```python
from build123d import *

# Parameters (mm, degrees)
F1_DEPTH    = 10
F2_R        = 1.5
F3_DEPTH    = 67.201
F5_DEPTH    = 1
F6_D        = 3.2
F7_R        = 4
F8_T1_DEPTH = 10


# Not quite as in the source:
# - a fillet or chamfer that OpenCascade refuses, or shapes differently, is made with other operations: its cross-section is extruded or revolved along the edge and cut away or added


with BuildPart() as f1:
    # F0 (on Front) → F1 (new body)
    with BuildSketch(Plane.XZ):
        with BuildLine():
            ThreePointArc((1, 29.5831032855), (0, -29.6), (-1, 29.5831032855))
            Line((-1, 29.5831032855), (-1, 41.225893517))
            Line((-1, 41.225893517), (-5, 41.225893517))
            Line((-5, 41.225893517), (-5, 33.225893517))
            ThreePointArc((-5, 33.225893517), (-19.3012329429, 27.503134492), (-29.5458965002, 16))
            Line((-29.5458965002, 16), (-33.6, 16))
            Line((-33.6, 16), (-33.6, -16))
            Line((-33.6, -16), (-29.5458965002, -16))
            ThreePointArc((-29.5458965002, -16), (0, -33.6), (29.5458965002, -16))
            Line((29.5458965002, -16), (33.6, -16))
            Line((33.6, -16), (33.6, 16))
            Line((33.6, 16), (29.5458965002, 16))
            ThreePointArc((29.5458965002, 16), (19.3012329429, 27.503134492), (5, 33.225893517))
            Line((5, 33.225893517), (5, 41.225893517))
            Line((5, 41.225893517), (1, 41.225893517))
            Line((1, 41.225893517), (1, 29.5831032855))
        make_face()
    extrude(amount=F1_DEPTH)

    # F2 (on face) → F3 (cut, through all)
    with BuildSketch(Plane.YZ.offset(33.6)):
        with Locations((-5, 10)):
            Circle(F2_R)
        with Locations((-5, -10)):
            Circle(F2_R)
    extrude(amount=-F3_DEPTH, mode=Mode.SUBTRACT)

    # F4 (on face) → F5 (cut)
    with BuildSketch(Plane.YZ.offset(5)):
        Polygon((-1.7091034656, 37.225893517), (-3.3545517328, 40.075893517), (-6.6454482672, 40.075893517), (-8.2908965344, 37.225893517), (-6.6454482672, 34.375893517), (-3.3545517328, 34.375893517), align=None)
    extrude(amount=-F5_DEPTH, mode=Mode.SUBTRACT)

    # F6 (through all)
    with Locations(Plane.YZ.offset(5)):
        with Locations((-5, 37.225893517)):
            Hole(F6_D / 2)

    # F7
    f7_edges = [f1.edges().sort_by_distance(p)[0] for p in [
        (3, 0, 41.225894),
        (3, -10, 41.225894),
        (-3, -10, 41.225894),
        (-3, 0, 41.225894),
    ]]
    fillet(f7_edges, radius=F7_R)

    # F8: chamfer of 1 on 2 edges, made by hand

    # F8_s2 → F8_t1 (join)
    with BuildSketch(Plane.XZ):
        with BuildLine():
            Line((4.9743446923, 34.2419704201), (5.9814730887, 33.0372447854))
            Line((5.9814730887, 33.0372447854), (5.977927959, 33.0175614916))
            ThreePointArc((5.977927959, 33.0175614916), (5.4901701774, 33.1281516451), (4.9970238095, 33.2061161994))
            Line((4.9970238095, 33.2061161994), (4.98, 33.225893517))
            ThreePointArc((4.98, 33.225893517), (4.98, 33.7339319685), (4.9543446923, 34.2419704201))
            Line((4.9543446923, 34.2419704201), (4.9743446923, 34.2419704201))
        make_face()
        with BuildLine():
            Line((-4.9743446923, 34.2419704201), (-5.9814730887, 33.0372447854))
            Line((-5.9814730887, 33.0372447854), (-5.977927959, 33.0175614916))
            ThreePointArc((-5.977927959, 33.0175614916), (-5.4901701774, 33.1281516451), (-4.9970238095, 33.2061161994))
            Line((-4.9970238095, 33.2061161994), (-4.98, 33.225893517))
            ThreePointArc((-4.98, 33.225893517), (-4.98, 33.7339319685), (-4.9543446923, 34.2419704201))
            Line((-4.9543446923, 34.2419704201), (-4.9743446923, 34.2419704201))
        make_face()
    extrude(amount=F8_T1_DEPTH)


solid = f1.part
```
The model under review builds one solid part; all positions refer to its coordinate system, in mm. A direction names the side the tool comes from. Coordinates: 2 decimals unless noted, no trailing zeros. Write each loop counter-clockwise with the first axis right and the second up, starting at its lowest first coordinate (ties: lowest second). Pieces come first, ordered by that corner, then holes.
1) We need section D-D on z = -10. State the section outline as (x, y) points, then the cut area to 3 significant figures.
2) Clearance check with flat-ended pins moving along their axes: pin 1 Ø2 at (x, y) = (-31, -5) entering from +Z; pin 2 Ø6 at (x, z) = (9, 24.5) entering from -Y; pin 3 Ø5 at (y, z) = (-5, 37.23) entering from -X; pin 4 Ø5 at (y, z) = (-8.5, 22) entering from +X. State where each tip first meets the part, or that it passes through.
3) We need section B-B on z = -23.5. State the section outline as (x, y) points.
4) We need section C-C on x = -23.5. State the section outline as (y, z) points, then the cut area to 3 significant figures.
5) To check wall thickness, follow probe 1 along Z at (x, y) = (30.5, -5); probe 2 along X at (y, z) = (-5.25, 35.5); probe 3 along Y at (x, z) = (-32, 10). State the ranges of each line that lie inside material, in increasing order.
6) Machinability: for faces 5 (the face through (4.51, -7.48, 35.82)), 6 (the face through (-5, -6, 39)), 7 (the face through (32, -5, -16)), 8 (the face through (-32, -5, -16)), which of the approach directions +Z, -Z, +X, -X, +Y, -Y give a long, thin tool a straight path to every point of the face, cutting with its end or side? Answer none if there is none.
7) We need section A-A on x = -2.5. State the section outline as (y, z) points.
8) The part is to be moulded in two halves that separate along X. For faces 1 (the face through (2.479, -5.738, 35.806)), 2 (the face through (5, -5, 41)), 3 (the face through (-1, -5, 35)), 4 (the face through (1.29, -4.93, -29.57)), say which applies: pulls with the +X half, pulls with the -X half, needs draft (parallel to the pull), parting line crosses it, or undercut.
Answer list:
1. outline: (-33.6, -10) - (-27.86, -10) - (-27.86, -6.5) - (-33.6, -6.5) - close; (-33.6, -3.5) - (-27.86, -3.5) - (-27.86, 0) - (-33.6, 0) - close; (27.86, -10) - (33.6, -10) - (33.6, -6.5) - (27.86, -6.5) - close; (27.86, -3.5) - (33.6, -3.5) - (33.6, 0) - (27.86, 0) - close
1. area: 80.4 mm2
2. pin 1: stops at z = 16
2. pin 2: passes through
2. pin 3: stops at x = -5
2. pin 4: stops at x = 27.36
3. outline: (-24.01, -10) - (-18, -10) - (-18, 0) - (-24.01, 0) - close; (18, -10) - (24.01, -10) - (24.01, 0) - (18, 0) - close
4. outline: (-10, -24.01) - (0, -24.01) - (0, -18) - (-10, -18) - close; (-10, 18) - (0, 18) - (0, 24.01) - (-10, 24.01) - close
4. area: 120 mm2
5. probe 1: z = -16 to -11.5, -8.5 to 8.5, 11.5 to 16
5. probe 2: x = -5 to -1, 1 to 4
5. probe 3: y = -10 to -6.5, -3.5 to 0
6. face 5: +X
6. face 6: +Z, -X, +Y, -Y
6. face 7: -Z, +X, +Y, -Y
6. face 8: -Z, -X, +Y, -Y
7. outline: (-10, -33.51) - (0, -33.51) - (0, -29.49) - (-10, -29.49) - close; (-10, 29.49) - (0, 29.49) - (0, 37.23) arc R4 ccw to (-4, 41.23) - (-6, 41.23) arc R4 ccw to (-10, 37.23) - close; hole circle Ø3.2 at (-5, 37.23)
8. face 1: needs draft
8. face 2: pulls with the +X half
8. face 3: undercut
8. face 4: undercut
